from build123d import *

# Parameters (mm, degrees)
F2_DEPTH = 89.8609068245
F3_R     = 39.4433228708
F4_DEPTH = 158.9131560177
F6_D     = 50.8


with BuildPart() as f2:
    # F0 (on Top) → F2 (new body)
    with BuildSketch(Plane.XY):
        Polygon((0, -106.1998531222), (0, 0), (-112.7292439342, 0), (-112.7292439342, -106.1998531222), (-56.3646219671, -106.1998531222), (-43.278105557, -106.1998531222), align=None)
    extrude(amount=F2_DEPTH)

    # F3 (on face) → F4 (join)
    with BuildSketch(Plane(origin=(0, 0, 0), x_dir=(-1, 0, 0), z_dir=(0, 1, 0))):
        with Locations((56.6163137555, 40.8002994955)):
            Circle(F3_R)
    extrude(amount=-F4_DEPTH)

    # F6 (through all)
    with Locations(Plane(origin=(0, 0, 0), x_dir=(1, 0, 0), z_dir=(0, 0, -1))):
        with Locations((-61.582095921, 53.7865236402)):
            Hole(F6_D / 2)


solid = f2.part
Model file for the job. Use its own axes, mm. A direction names the side the tool comes from. Coordinates: 2 decimals unless noted, no trailing zeros. Loops run counter-clockwise (first coordinate to the right, second up) from the corner with the lowest first, then second, coordinate; pieces in that order, holes last. Notation, with made-up numbers: (66, 29) -> (85, 29) arc R6 ccw to (85, 36) -> close; hole circle Ø6 at (-37, 72.5). An arc over 180 degrees is marked (long way). Use one line per item in the form item = value. Start each with the question number.
(1) Tool access for faces 4 (the flat face through (-82, -106.2, 74)), 5 (the flat face through (0, -54, 44)): list every direction of +Z, -Z, +X, -X, +Y, -Y with a clear straight run to the whole face (end or side of a thin tool).
(2) Cut at D-D on x = -31.5. Give the cut face in (y, z), and give its area (3 significant figures).
(3) Flat gauge pins, fed straight in: pin 1 (4 mm diameter, centred on x = -34, y = -141.5, fed in from -Z); pin 2 (4 mm diameter, centred on x = -58.5, z = 24.5, fed in from +Y); pin 3 (1 mm diameter, centred on y = -113.5, z = 23, fed in from +X); pin 4 (5 mm diameter, centred on x = -93.5, z = 70.5, fed in from -Y). Where does each tip first touch, or does it go through?
(4) Cut at C-C on x = -67. Give the cut face in (y, z), and give its area (3 significant figures).
(5) Cut at B-B on z = 13.5. Give the cut face in (x, y), and give its area (3 significant figures).
(6) Pull direction Y, two halves, no side cores. Call faces 1 (the cylindrical face through (-48.066, -132.188, 2.295)), 2 (the flat face through (-56, -158.913, 41)), 3 (the cylindrical face through (-73.3, -31.25, 45.56)): pulls with the +Y half, pulls with the -Y half, needs draft (parallel to the pull), parting line crosses it, or undercut.
(7) Probe probe 1 along Y at (x, z) = (-101.5, 70); probe 2 along X at (y, z) = (-67, 44); probe 3 along X at (y, z) = (-36, 13.5). List the from-to ranges inside material, lowest first. Write a range as from..to.
(8) Cut at A-A on y = -56. Give the cut face in (x, z), and give its area (3 significant figures).
Values:
q1.face_4 = -Y
q1.face_5 = +Z, -Z, +X, +Y, -Y
q2.outline = (-158.91, 10.39) -> (-106.2, 10.39) -> (-106.2, 0) -> (0, 0) -> (0, 89.86) -> (-106.2, 89.86) -> (-106.2, 71.21) -> (-158.91, 71.21) -> close
q2.area = 12,700 mm2
q3.pin_1 = 7.17
q3.pin_2 = 0
q3.pin_3 = -21.17
q3.pin_4 = -106.2
q4.outline = (-158.91, 2.75) -> (-106.2, 2.75) -> (-106.2, 0) -> (-78.6, 0) -> (-78.6, 89.86) -> (-106.2, 89.86) -> (-106.2, 78.85) -> (-158.91, 78.85) -> close; (-28.97, 0) -> (0, 0) -> (0, 89.86) -> (-28.97, 89.86) -> close
q4.area = 9,100 mm2
q5.outline = (-112.73, -106.2) -> (-85.09, -106.2) -> (-85.09, -158.91) -> (-28.15, -158.91) -> (-28.15, -106.2) -> (0, -106.2) -> (0, 0) -> (-112.73, 0) -> close; hole circle Ø50.8 at (-61.58, -53.79)
q5.area = 12,900 mm2
q6.face_1 = needs draft
q6.face_2 = pulls with the -Y half
q6.face_3 = undercut
q7.probe_1 = -106.2..0
q7.probe_2 = -112.73..-83.27, -39.89..0
q7.probe_3 = -112.73..-79.71, -43.45..0
q8.outline = (-112.73, 0) -> (-86.89, 0) -> (-86.89, 89.86) -> (-112.73, 89.86) -> close; (-36.28, 0) -> (0, 0) -> (0, 89.86) -> (-36.28, 89.86) -> close
q8.area = 5,580 mm2
